Autodesk Inventor part; units mm, degrees
ref_plane "YZ Plane" through (0, 0, 0) normal (1, 0, 0) x (0, 1, 0)
ref_plane "XZ Plane" through (0, 0, 0) normal (0, 1, 0) x (-1, 0, 0)
ref_plane "XY Plane" through (0, 0, 0) normal (0, 0, 1) x (1, 0, 0)
sketch "Sketch2" plane through (0, 0, 0) normal (0, 1, 0) x (-1, 0, 0)
  line L0 (0, 0) -> (-60, 0)
  line L1 (-60, 0) -> (-60, -38)
  line L2 (-60, -38) -> (0, -38)
  line L3 (0, -38) -> (0, 0)
  dimension "d2" = 60
  dimension "d3" = 38
extrude "Extrusion1" add sketch "Sketch2" along normal blind 5
sketch "Sketch3" plane through (0, 0, 0) normal (0, -1, 0) x (1, 0, 0)
  line L0 (55, -32) -> (5, -32)
  line L1 (5, -32) -> (5, -12)
  line L2 (5, -12) -> (55, -12)
  line L3 (55, -12) -> (55, -32)
  line L4 (60, -38) -> (0, -38)
  line L5 (60, 0) -> (60, -38)
  point P0 (0, 0)
  dimension "d6" = 50
  dimension "d7" = 20
  dimension "d8" = 6
  dimension "d9" = 5
extrude "Extrusion2" cut sketch "Sketch3" against normal blind 2
sketch "Sketch5" plane through (0, 0, 0) normal (0, -1, 0) x (1, 0, 0)
  circle A0 centre (58, -36) radius 1.5
  line L0 (60, 0) -> (60, -38)
  line L1 (60, -38) -> (0, -38)
  line L2 (0, -38) -> (0, 0)
  dimension "d14" = 3
  dimension "d15" = 2
  dimension "d16" = 2
extrude "Extrusion3" cut sketch "Sketch5" against normal blind 5
sketch "Sketch6" plane through (0, 0, 0) normal (0, -1, 0) x (1, 0, 0)
  circle A0 centre (53, -3) radius 1.5
  line L0 (60, 0) -> (60, -38)
  line L1 (0, 0) -> (60, 0)
  circle A1 centre (7, -3) radius 1.5
  line L2 (0, -38) -> (0, 0)
  dimension "d22" = 3
  dimension "d23" = 7
  dimension "d24" = 3
  dimension "d25" = 3
  dimension "d26" = 7
  dimension "d27" = 3
extrude "Extrusion4" cut sketch "Sketch6" against normal blind 5
sketch "Sketch7" plane through (0, 5, 0) normal (0, 1, 0) x (1, 0, 0)
  line L0 (0, 38) -> (0, 0)
  line L1 (0, 38) -> (4, 38)
  line L2 (4, 38) -> (4, 16.5)
  line L3 (4, 16.5) -> (0, 16.5)
  line L4 (0, 16.5) -> (0, 38)
  dimension "d36" = 4
  dimension "d37" = 21.5
extrude "Extrusion5" cut sketch "Sketch7" against normal blind 10
sketch "Sketch8" plane through (0, 5, 0) normal (0, 1, 0) x (1, 0, 0)
  circle A0 centre (6, 36) radius 1.5
  line L0 (4, 38) -> (4, 16.5)
  line L1 (60, 38) -> (4, 38)
  point P0 (0, 0)
  dimension "d40" = 3
  dimension "d41" = 2
  dimension "d42" = 2
extrude "Extrusion6" cut sketch "Sketch8" against normal blind 10
properties part number "PiBed"
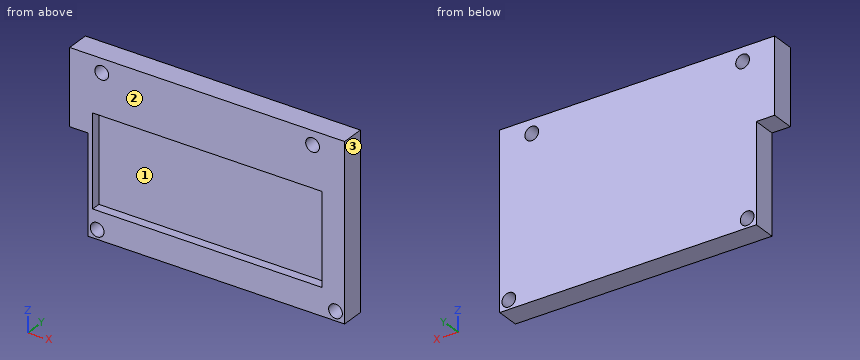
Part model, mm, in its own coordinate system. Face numbers are marked on the shaded views. Round coordinates to 2 decimals unless told otherwise and drop trailing zeros. Loops run counter-clockwise (first coordinate to the right, second up) from the corner with the lowest first, then second, coordinate; pieces in that order, holes last.
Item 1: Cut at C-C, the plane y = 3.55. Give the cut face in (x, z).
Item 2: Cut at D-D, the plane z = -27.5. Give the cut face in (x, y).
Item 3: Drill centre lines: line 1 (X direction, y = 0.45, z = -22); line 2 (Z direction, x = 15.5, y = 1.5); line 3 (X direction, y = 2.35, z = -28). Where is each one in solid material? Low to high.
Item 4: Mould opens along X. For the marked faces 1, 2 and 3 say: +X half, -X half, draft (parallel to the pull), parting line (faces both ways), or undercut.
Item 5: Cut at B-B, the plane x = 53. Give the cut face in (y, z).
Item 6: Cut at A-A, the plane z = -3. Give the cut face in (x, y), then the cut area to 3 significant figures.
Item 7: Drop flat-ended pins along their axis: P1, Ø2.5, axis at x = 6, z = -36, coming from the +Y side; P2, Ø10, axis at x = 17.5, z = -18, coming from the -Y side; P3, Ø4, axis at x = 58, z = -36, coming from the +Y side; P4, Ø1.2, axis at x = 1.5, y = 2.5, coming from the -Z side. Give the stop position or say it passes through.
A:
1. outline: (0, -16.5) - (4, -16.5) - (4, -38) - (60, -38) - (60, 0) - (0, 0) - close; hole circle Ø3 at (6, -36); hole circle Ø3 at (7, -3); hole circle Ø3 at (53, -3); hole circle Ø3 at (58, -36)
2. outline: (4, 0) - (5, 0) - (5, 2) - (55, 2) - (55, 0) - (60, 0) - (60, 5) - (4, 5) - close
3. line 1: x = 4 to 5, 55 to 60
3. line 2: z = -38 to -32, -12 to 0
3. line 3: x = 4 to 60
4. face 1: undercut
4. face 2: draft
4. face 3: +X half
5. outline: (0, -38) - (5, -38) - (5, -4.5) - (0, -4.5) - (0, -12) - (2, -12) - (2, -32) - (0, -32) - close; (0, -1.5) - (5, -1.5) - (5, 0) - (0, 0) - close
6. outline: (0, 0) - (5.5, 0) - (5.5, 5) - (0, 5) - close; (8.5, 0) - (51.5, 0) - (51.5, 5) - (8.5, 5) - close; (54.5, 0) - (60, 0) - (60, 5) - (54.5, 5) - close
6. area: 270 mm2
7. P1: passes through
7. P2: stops at y = 2
7. P3: stops at y = 5
7. P4: stops at z = -16.5
